```python
from build123d import *

# Parameters (mm, degrees)
BOSS_EXTRUDE1_START     = 5.08
BOSS_EXTRUDE1_DEPTH     = 43.18
SKETCH2_W               = 51
SKETCH2_H               = 8.231998532
BOSS_EXTRUDE2_DEPTH     = 5.08
CUT_EXTRUDE1_DEPTH      = 100.957396182
CUT_EXTRUDE1_DEPTH_BACK = 5.08
SKETCH3_R               = 1.05
SKETCH4_R               = 1.25
CUT_EXTRUDE2_DEPTH      = 5.08
SKETCH5_W               = 51
SKETCH5_H               = 8.231998532
BOSS_EXTRUDE3_DEPTH     = 5.08
BOSS_EXTRUDE4_DEPTH     = 5.08
FILLET1_R               = 2.54
SKETCH7_W               = 75.202673557
SKETCH7_H               = 41.660019182
CUT_EXTRUDE3_DEPTH      = 80.950255842


with BuildPart() as part:
    # Sketch1 → Boss-Extrude1 (new body)
    with BuildSketch(Plane.XY.offset(58.730428606).offset(BOSS_EXTRUDE1_START)):
        Polygon((-14.213699035, 28.595837466), (-14.213699035, 47.595837466), (36.786300965, 47.595837466), (36.786300965, 28.595837466), (41.866300965, 28.595837466), (41.866300965, 52.675837466), (-19.293699035, 52.675837466), (-19.293699035, 28.595837466), align=None)
    extrude(amount=-BOSS_EXTRUDE1_DEPTH)

    # Sketch2 → Boss-Extrude2 (add)
    with BuildSketch(Plane(origin=(0, 0, 20.630428606), x_dir=(-1, 0, 0), z_dir=(0, 0, -1))):
        with Locations((-11.286300965, 43.4798382)):
            Rectangle(SKETCH2_W, SKETCH2_H)
    extrude(amount=-BOSS_EXTRUDE2_DEPTH)

    # Sketch3 → Cut-Extrude1 (cut, two sides: drawn at the far end of the back side and taken through both)
    with BuildSketch(Plane.ZY.offset(-36.786300965).offset(-CUT_EXTRUDE1_DEPTH_BACK)):
        with Locations(Location((50.230428606, 32.595837466, 0), (0, 0, 180))):
            Circle(SKETCH3_R)
        with Locations(Location((34.230428606, 32.595837466, 0), (0, 0, 180))):
            Circle(SKETCH3_R)
    extrude(amount=CUT_EXTRUDE1_DEPTH + CUT_EXTRUDE1_DEPTH_BACK, mode=Mode.SUBTRACT)

    # Sketch4 → Cut-Extrude2 (cut)
    with BuildSketch(Plane(origin=(0, 47.595837466, 0), x_dir=(-1, 0, 0), z_dir=(0, -1, 0))):
        with Locations(Location((-22.286300965, -42.230428606, 0), (0, 0, 90))):
            Circle(SKETCH4_R)
        with Locations(Location((-11.286300965, -53.230428606, 0), (0, 0, 90))):
            Circle(SKETCH4_R)
        with Locations(Location((-11.286300965, -31.230428606, 0), (0, 0, 90))):
            Circle(SKETCH4_R)
        with Locations(Location((-0.286300965, -42.230428606, 0), (0, 0, 90))):
            Circle(SKETCH4_R)
    extrude(amount=-CUT_EXTRUDE2_DEPTH, mode=Mode.SUBTRACT)

    # Sketch5 → Boss-Extrude3 (add)
    with BuildSketch(Plane.XY.offset(63.810428606)):
        with Locations((11.286300965, 43.4798382)):
            Rectangle(SKETCH5_W, SKETCH5_H)
    extrude(amount=-BOSS_EXTRUDE3_DEPTH)

    # Sketch6 → Boss-Extrude4 (add)
    with BuildSketch(Plane.ZY.offset(19.293699035)):
        with BuildLine():
            Line((63.810428606, 28.595837466), (20.630428606, 28.595837466))
            Line((20.630428606, 28.595837466), (20.630428606, 11.595837466))
            Line((20.630428606, 11.595837466), (28.120807374, 11.595837466))
            ThreePointArc((28.120807374, 11.595837466), (42.230428606, 25.705458697), (56.340049838, 11.595837466))
            Line((56.340049838, 11.595837466), (63.810428606, 11.595837466))
            Line((63.810428606, 11.595837466), (63.810428606, 28.595837466))
        make_face()
    extrude(amount=-BOSS_EXTRUDE4_DEPTH)

    # Fillet1
    fillet1_edges = [part.edges().sort_by_distance(p)[0] for p in [
        (41.866300965, 52.675837466, 42.220428606),
        (39.326300965, 28.595837466, 20.630428606),
        (11.286300965, 52.675837466, 20.630428606),
        (-14.213699035, 39.363838934, 23.170428606),
        (-14.213699035, 39.363838934, 61.270428606),
        (11.286300965, 52.675837466, 63.810428606),
        (39.326300965, 28.595837466, 63.810428606),
    ]]
    fillet(fillet1_edges, radius=FILLET1_R)

    # Sketch7 → Cut-Extrude3 (cut, through all)
    with BuildSketch(Plane.XY.offset(63.810428606)):
        with Locations((23.387637744, 39.269623894)):
            Rectangle(SKETCH7_W, SKETCH7_H)
    extrude(amount=-CUT_EXTRUDE3_DEPTH, mode=Mode.SUBTRACT)


solid = part.part
```
The model under review builds one solid part; all positions refer to its coordinate system, in mm. Round coordinates to 2 decimals unless told otherwise and drop trailing zeros. Write each loop counter-clockwise with the first axis right and the second up, starting at its lowest first coordinate (ties: lowest second). Pieces come first, ordered by that corner, then holes. Notation, with made-up numbers: (78, 16.25) - (129, 16.25) arc R10 cw to (129, 22.25) - close; hole circle Ø8 at (-37, -14). An arc over 180 degrees is marked (long way). Answer as CSV lines item,"result". Start each with the question number.
(1) We need section A-A on y = 21.5. State the section outline as (x, z) points, plus the area to 3 significant figures.
(2) We need section D-D on z = 43. State the section outline as (x, y) points.
(3) To check wall thickness, follow line 1 (Z direction, x = -16.55, y = 32) (3 decimals); line 2 (Z direction, x = -16.5, y = 33); line 3 (Z direction, x = -14.6, y = 20.5). State the ranges of each line that lie inside material, in increasing order.
(4) We need section B-B on x = -18.05. State the section outline as (y, z) points, plus the area to 3 significant figures.
(5) Draft analysis for pull direction Z (two halves, no side actions). For faces 1 (the flat face through (-17, 11.596, 24)), 2 (the cylindrical face through (-16.72, 31.71, 33.67)), 3 (the flat face through (-17, 31, 63.81)), state which applies: pulls with the +Z half, pulls with the -Z half, needs draft (parallel to the pull), parting line crosses it, or undercut.
(6) We need section C-C on z = 36.5. State the section outline as (x, y) points.
Worked answers:
1,outline,"(-19.29, 20.63) - (-14.21, 20.63) - (-14.21, 32.18) - (-19.29, 32.18) - close; (-19.29, 52.28) - (-14.21, 52.28) - (-14.21, 63.81) - (-19.29, 63.81) - close"
1,area,"117 mm²"
2,outline,"(-19.29, 25.68) - (-14.21, 25.68) - (-14.21, 52.68) - (-19.29, 52.68) - close"
3,line 1,"20.63 to 33.366, 35.095 to 49.366, 51.095 to 63.81"
3,line 2,"20.63 to 33.26, 35.2 to 49.26, 51.2 to 63.81"
3,line 3,"20.63 to 31.29, 53.18 to 63.81"
4,outline,"(11.6, 20.63) - (50.14, 20.63) arc R2.54 ccw to (52.68, 23.17) - (52.68, 61.27) arc R2.54 ccw to (50.14, 63.81) - (11.6, 63.81) - (11.6, 56.34) arc R14.11 cw to (11.6, 28.12) - close; hole circle Ø2.1 at (32.6, 34.23); hole circle Ø2.1 at (32.6, 50.23)"
4,area,"1,450 mm²"
5,face 1,"needs draft"
5,face 2,"undercut"
5,face 3,"pulls with the +Z half"
6,outline,"(-19.29, 24.49) - (-14.21, 24.49) - (-14.21, 52.68) - (-19.29, 52.68) - close"
